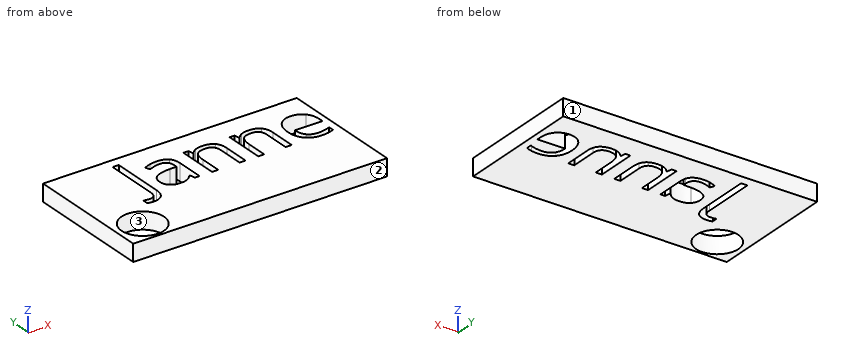
from build123d import *

# Parameters (mm, degrees)
F0_W     = 30
F0_H     = 15
F1_DEPTH = 2
F3_D     = 5
F3_DEPTH = 2
F3_TIP   = 1.5021515476


with BuildPart() as f1:
    # F0 (on Top) → F1 (new body)
    with BuildSketch(Plane.XY):
        with Locations((-15, 7.5)):
            Rectangle(F0_W, F0_H)
        with BuildLine():
            add(Edge.make_bspline(
                [(-22.2773678395, 6.2837986352), (-22.6936375593, 5.8307584235), (-23.4748370669, 5.8307584235)],
                knots=[0, 0, 0, 1, 1, 1], degree=2))
            add(Edge.make_bspline(
                [(-23.4748370669, 5.8307584235), (-23.8813938266, 5.8307584235), (-24.1158924354, 5.947313945)],
                knots=[0, 0, 0, 1, 1, 1], degree=2))
            Line((-24.1158924354, 5.947313945), (-24.1158924354, 6.575881222))
            add(Edge.make_bspline(
                [(-24.1158924354, 6.575881222), (-23.8078528427, 6.4898521465), (-23.4748370669, 6.4898521465)],
                knots=[0, 0, 0, 1, 1, 1], degree=2))
            add(Edge.make_bspline(
                [(-23.4748370669, 6.4898521465), (-23.0446916897, 6.4898521465), (-22.8212936067, 6.7500207214)],
                knots=[0, 0, 0, 1, 1, 1], degree=2))
            add(Edge.make_bspline(
                [(-22.8212936067, 6.7500207214), (-22.5978955238, 7.0101892963), (-22.5978955238, 7.5)],
                knots=[0, 0, 0, 1, 1, 1], degree=2))
            Line((-22.5978955238, 7.5), (-22.5978955238, 13.839787833))
            Line((-22.5978955238, 13.839787833), (-21.8610981197, 13.839787833))
            Line((-21.8610981197, 13.839787833), (-21.8610981197, 7.5610528922))
            add(Edge.make_bspline(
                [(-21.8610981197, 7.5610528922), (-21.8610981197, 6.736838847), (-22.2773678395, 6.2837986352)],
                knots=[0, 0, 0, 1, 1, 1], degree=2))
        make_face(mode=Mode.SUBTRACT)
        with BuildLine():
            Line((-16.8311723384, 7.5), (-17.3653851455, 7.5))
            Line((-17.3653851455, 7.5), (-17.508304416, 8.1771320776))
            Line((-17.508304416, 8.1771320776), (-17.5429935593, 8.1771320776))
            add(Edge.make_bspline(
                [(-17.5429935593, 8.1771320776), (-17.8982103869, 7.7303359116), (-18.2513458659, 7.5714596352)],
                knots=[0, 0, 0, 1, 1, 1], degree=2))
            add(Edge.make_bspline(
                [(-18.2513458659, 7.5714596352), (-18.6044813449, 7.4125833588), (-19.1345314548, 7.4125833588)],
                knots=[0, 0, 0, 1, 1, 1], degree=2))
            add(Edge.make_bspline(
                [(-19.1345314548, 7.4125833588), (-19.8408024128, 7.4125833588), (-20.2418089095, 7.7775131466)],
                knots=[0, 0, 0, 1, 1, 1], degree=2))
            add(Edge.make_bspline(
                [(-20.2418089095, 7.7775131466), (-20.6428154063, 8.1424429343), (-20.6428154063, 8.8140247489)],
                knots=[0, 0, 0, 1, 1, 1], degree=2))
            add(Edge.make_bspline(
                [(-20.6428154063, 8.8140247489), (-20.6428154063, 10.2529304138), (-18.3408438557, 10.3223087004)],
                knots=[0, 0, 0, 1, 1, 1], degree=2))
            Line((-18.3408438557, 10.3223087004), (-17.5346681649, 10.3486724494))
            Line((-17.5346681649, 10.3486724494), (-17.5346681649, 10.6442239504))
            add(Edge.make_bspline(
                [(-17.5346681649, 10.6442239504), (-17.5346681649, 11.2034129407), (-17.7747170367, 11.4698255614)],
                knots=[0, 0, 0, 1, 1, 1], degree=2))
            add(Edge.make_bspline(
                [(-17.7747170367, 11.4698255614), (-18.0147659085, 11.7362381821), (-18.5448160184, 11.7362381821)],
                knots=[0, 0, 0, 1, 1, 1], degree=2))
            add(Edge.make_bspline(
                [(-18.5448160184, 11.7362381821), (-19.138694152, 11.7362381821), (-19.8879796477, 11.3726959601)],
                knots=[0, 0, 0, 1, 1, 1], degree=2))
            Line((-19.8879796477, 11.3726959601), (-20.1099901649, 11.923559556))
            add(Edge.make_bspline(
                [(-20.1099901649, 11.923559556), (-19.7589360345, 12.1136560614), (-19.3405849661, 12.2218861886)],
                knots=[0, 0, 0, 1, 1, 1], degree=2))
            add(Edge.make_bspline(
                [(-19.3405849661, 12.2218861886), (-18.9222338977, 12.3301163157), (-18.5004139149, 12.3301163157)],
                knots=[0, 0, 0, 1, 1, 1], degree=2))
            add(Edge.make_bspline(
                [(-18.5004139149, 12.3301163157), (-17.6512236865, 12.3301163157), (-17.2411980124, 11.9533922193)],
                knots=[0, 0, 0, 1, 1, 1], degree=2))
            add(Edge.make_bspline(
                [(-17.2411980124, 11.9533922193), (-16.8311723384, 11.5766681229), (-16.8311723384, 10.7441286832)],
                knots=[0, 0, 0, 1, 1, 1], degree=2))
            Line((-16.8311723384, 10.7441286832), (-16.8311723384, 7.5))
        make_face(mode=Mode.SUBTRACT)
        with BuildLine():
            Line((-11.3766514429, 7.5), (-12.0967980582, 7.5))
            Line((-12.0967980582, 7.5), (-12.0967980582, 10.5748456638))
            add(Edge.make_bspline(
                [(-12.0967980582, 10.5748456638), (-12.0967980582, 11.1548481401), (-12.3611293303, 11.4413804639)],
                knots=[0, 0, 0, 1, 1, 1], degree=2))
            add(Edge.make_bspline(
                [(-12.3611293303, 11.4413804639), (-12.6254606024, 11.7279127877), (-13.1901998556, 11.7279127877)],
                knots=[0, 0, 0, 1, 1, 1], degree=2))
            add(Edge.make_bspline(
                [(-13.1901998556, 11.7279127877), (-13.9353226541, 11.7279127877), (-14.2822140873, 11.3248249424)],
                knots=[0, 0, 0, 1, 1, 1], degree=2))
            add(Edge.make_bspline(
                [(-14.2822140873, 11.3248249424), (-14.6291055205, 10.921737097), (-14.6291055205, 9.9934556218)],
                knots=[0, 0, 0, 1, 1, 1], degree=2))
            Line((-14.6291055205, 9.9934556218), (-14.6291055205, 7.5))
            Line((-14.6291055205, 7.5), (-15.3492521358, 7.5))
            Line((-15.3492521358, 7.5), (-15.3492521358, 12.2524126347))
            Line((-15.3492521358, 12.2524126347), (-14.7636993966, 12.2524126347))
            Line((-14.7636993966, 12.2524126347), (-14.647143875, 11.601644306))
            Line((-14.647143875, 11.601644306), (-14.6124547317, 11.601644306))
            add(Edge.make_bspline(
                [(-14.6124547317, 11.601644306), (-14.3904442145, 11.9526984364), (-13.9915190663, 12.1462638562)],
                knots=[0, 0, 0, 1, 1, 1], degree=2))
            add(Edge.make_bspline(
                [(-13.9915190663, 12.1462638562), (-13.5925939181, 12.3398292759), (-13.1027832145, 12.3398292759)],
                knots=[0, 0, 0, 1, 1, 1], degree=2))
            add(Edge.make_bspline(
                [(-13.1027832145, 12.3398292759), (-12.2438800259, 12.3398292759), (-11.8102657344, 11.9256409046)],
                knots=[0, 0, 0, 1, 1, 1], degree=2))
            add(Edge.make_bspline(
                [(-11.8102657344, 11.9256409046), (-11.3766514429, 11.5114525334), (-11.3766514429, 10.599821847)],
                knots=[0, 0, 0, 1, 1, 1], degree=2))
            Line((-11.3766514429, 10.599821847), (-11.3766514429, 7.5))
        make_face(mode=Mode.SUBTRACT)
        with BuildLine():
            Line((-5.9262932446, 7.5), (-6.6464398599, 7.5))
            Line((-6.6464398599, 7.5), (-6.6464398599, 10.5748456638))
            add(Edge.make_bspline(
                [(-6.6464398599, 10.5748456638), (-6.6464398599, 11.1548481401), (-6.910771132, 11.4413804639)],
                knots=[0, 0, 0, 1, 1, 1], degree=2))
            add(Edge.make_bspline(
                [(-6.910771132, 11.4413804639), (-7.1751024041, 11.7279127877), (-7.7398416573, 11.7279127877)],
                knots=[0, 0, 0, 1, 1, 1], degree=2))
            add(Edge.make_bspline(
                [(-7.7398416573, 11.7279127877), (-8.4849644558, 11.7279127877), (-8.831855889, 11.3248249424)],
                knots=[0, 0, 0, 1, 1, 1], degree=2))
            add(Edge.make_bspline(
                [(-8.831855889, 11.3248249424), (-9.1787473222, 10.921737097), (-9.1787473222, 9.9934556218)],
                knots=[0, 0, 0, 1, 1, 1], degree=2))
            Line((-9.1787473222, 9.9934556218), (-9.1787473222, 7.5))
            Line((-9.1787473222, 7.5), (-9.8988939375, 7.5))
            Line((-9.8988939375, 7.5), (-9.8988939375, 12.2524126347))
            Line((-9.8988939375, 12.2524126347), (-9.3133411983, 12.2524126347))
            Line((-9.3133411983, 12.2524126347), (-9.1967856767, 11.601644306))
            Line((-9.1967856767, 11.601644306), (-9.1620965334, 11.601644306))
            add(Edge.make_bspline(
                [(-9.1620965334, 11.601644306), (-8.9400860162, 11.9526984364), (-8.541160868, 12.1462638562)],
                knots=[0, 0, 0, 1, 1, 1], degree=2))
            add(Edge.make_bspline(
                [(-8.541160868, 12.1462638562), (-8.1422357198, 12.3398292759), (-7.6524250162, 12.3398292759)],
                knots=[0, 0, 0, 1, 1, 1], degree=2))
            add(Edge.make_bspline(
                [(-7.6524250162, 12.3398292759), (-6.7935218276, 12.3398292759), (-6.3599075361, 11.9256409046)],
                knots=[0, 0, 0, 1, 1, 1], degree=2))
            add(Edge.make_bspline(
                [(-6.3599075361, 11.9256409046), (-5.9262932446, 11.5114525334), (-5.9262932446, 10.599821847)],
                knots=[0, 0, 0, 1, 1, 1], degree=2))
            Line((-5.9262932446, 10.599821847), (-5.9262932446, 7.5))
        make_face(mode=Mode.SUBTRACT)
        with BuildLine():
            add(Edge.make_bspline(
                [(-1.6192892101, 7.4847367769), (-1.9592428147, 7.4125833588), (-2.4407281239, 7.4125833588)],
                knots=[0, 0, 0, 1, 1, 1], degree=2))
            add(Edge.make_bspline(
                [(-2.4407281239, 7.4125833588), (-3.4938905151, 7.4125833588), (-4.1037256546, 8.0550262931)],
                knots=[0, 0, 0, 1, 1, 1], degree=2))
            add(Edge.make_bspline(
                [(-4.1037256546, 8.0550262931), (-4.7135607942, 8.6974692274), (-4.7135607942, 9.836660694)],
                knots=[0, 0, 0, 1, 1, 1], degree=2))
            add(Edge.make_bspline(
                [(-4.7135607942, 9.836660694), (-4.7135607942, 10.9869526864), (-4.1474339752, 11.6633909812)],
                knots=[0, 0, 0, 1, 1, 1], degree=2))
            add(Edge.make_bspline(
                [(-4.1474339752, 11.6633909812), (-3.5813071563, 12.3398292759), (-2.6266619321, 12.3398292759)],
                knots=[0, 0, 0, 1, 1, 1], degree=2))
            add(Edge.make_bspline(
                [(-2.6266619321, 12.3398292759), (-1.734457166, 12.3398292759), (-1.2141200162, 11.752195188)],
                knots=[0, 0, 0, 1, 1, 1], degree=2))
            add(Edge.make_bspline(
                [(-1.2141200162, 11.752195188), (-0.6937828664, 11.1645611002), (-0.6937828664, 10.2015904817)],
                knots=[0, 0, 0, 1, 1, 1], degree=2))
            Line((-0.6937828664, 10.2015904817), (-0.6937828664, 9.7464689213))
            Line((-0.6937828664, 9.7464689213), (-3.96705043, 9.7464689213))
            add(Edge.make_bspline(
                [(-3.96705043, 9.7464689213), (-3.9448493782, 8.9097667845), (-3.5438428815, 8.476152493)],
                knots=[0, 0, 0, 1, 1, 1], degree=2))
            add(Edge.make_bspline(
                [(-3.5438428815, 8.476152493), (-3.1428363847, 8.0425382015), (-2.414364375, 8.0425382015)],
                knots=[0, 0, 0, 1, 1, 1], degree=2))
            add(Edge.make_bspline(
                [(-2.414364375, 8.0425382015), (-1.6470405248, 8.0425382015), (-0.8977550291, 8.3630658858)],
                knots=[0, 0, 0, 1, 1, 1], degree=2))
            Line((-0.8977550291, 8.3630658858), (-0.8977550291, 7.7206229515))
            add(Edge.make_bspline(
                [(-0.8977550291, 7.7206229515), (-1.2793356056, 7.556890195), (-1.6192892101, 7.4847367769)],
                knots=[0, 0, 0, 1, 1, 1], degree=2))
        make_face(mode=Mode.SUBTRACT)
    extrude(amount=-F1_DEPTH)

    # F3
    with Locations(Plane.XY):
        with Locations((-26.8938727677, 2.7855671942)):
            Hole(F3_D / 2, depth=F3_DEPTH)
            with Locations((0, 0, -(F3_DEPTH + F3_TIP / 2))):  # 118° drill point
                Cone(0, F3_D / 2, F3_TIP, mode=Mode.SUBTRACT)


solid = f1.part
Here's how the part is built. I have some questions about the finished solid (model axes, mm). Face numbers are marked on the shaded views. Give positions to 0.01 mm unless a question says otherwise; leave off trailing zeros. Write each loop counter-clockwise with the first axis right and the second up, starting at its lowest first coordinate (ties: lowest second). Pieces come first, ordered by that corner, then holes. Notation, with made-up numbers: (46, 76) -> (97, 76) arc R15 ccw to (97, 101) -> close; hole circle Ø4 at (-7, 67.25). An arc over 180 degrees is marked (long way). Use one line per item in the form item = value. Start each with the question number.
1. Will this pin go through, and if not, where does the flat tip stop? pin 1 Ø1 at (y, z) = (8.5, -0.5) entering from +X.
2. If I drill on L1, parallel to Y at x = -2.5, z = -0.05; L2, parallel to X at y = 12.5, z = -1.5; L3, parallel to Y at x = -15, z = -1.75, over which ranges is the centre line in solid material (lowest first)?
3. Imagine slicing it at C-C on z = -1.25. State how many separate pieces and enclosed holes the cut face has, plus the area to 3 significant figures.
4. Imagine slicing it at A-A on y = 4.25. List the corners of the cut face in (x, z) for me, plus the area to 3 significant figures.
5. Imagine slicing it at B-B on x = -26. List the corners of the cut face in (y, z) for me.
6. Thinking about a two-plate mould opening in Y: for the marked faces 1, 2 and 3, which applies, +Y half, -Y half, draft (parallel to the pull), parting line (faces both ways), or undercut?
Entries:
q1.pin_1 = 0
q2.L1 = 0 to 7.41, 8.04 to 9.75, 12.34 to 15
q2.L2 = -30 to -22.6, -21.86 to 0
q2.L3 = 0 to 7.5, 12.25 to 15
q3.separate_pieces = 1
q3.enclosed_holes = 6
q3.area = 383 mm²
q4.outline = (-30, -2) -> (-28.92, -2) -> (-28.92, 0) -> (-30, 0) -> close; (-24.87, -2) -> (0, -2) -> (0, 0) -> (-24.87, 0) -> close
q4.area = 51.9 mm²
q5.outline = (0, -2) -> (0.45, -2) -> (0.45, 0) -> (0, 0) -> close; (5.12, -2) -> (15, -2) -> (15, 0) -> (5.12, 0) -> close
q6.face_1 = +Y half
q6.face_2 = -Y half
q6.face_3 = undercut
